The figure shows three views and two pictorial views of one solid part (mm, origin at its lowest corner). Answer the questions. Coordinates: 2 decimals unless noted, no trailing zeros. Order: outer loops, then holes, each group sorted by start corner. A loop starts at its lowest first (then second) coordinate and runs counter-clockwise, first axis right, second up. Notation, with made-up numbers: M -37.75,19.25 L 13.25,19.25 A14 ccw 13.25,33.25 Z; hole C 37,21 d9. An arc over 180 degrees is marked long. Write item = value, one per line. Start each with the question number.
Q1. Find section A-A on z = 3.25. Give the vertices of the cut face in (x, y), and give its area (3 significant figures).
Q2. Straight lines are drawn through the part: line 1 along Y through (x, z) = (36, 11.5); line 2 along X through (y, z) = (64.5, 9.25); line 3 along Y through (x, z) = (5, 7). For each, find the intervals that lie inside material, in ascending order.
Q3. Each of these flat-tipped pins is pushed along its axis until it touches: P1, Ø3, axis at y = 32.5, z = 20.5, coming from the -X side; P2, Ø2, axis at x = 54.5, z = 10.5, coming from the -Y side; P3, Ø4, axis at y = 58.5, z = 8, coming from the -X side. Where does it stop, or does it pass through?
Q4. Determine the mould class of the marked faces 1 and 2 for opening direction X: released by +X, released by -X, zero draft, split by the parting line, or undercut.
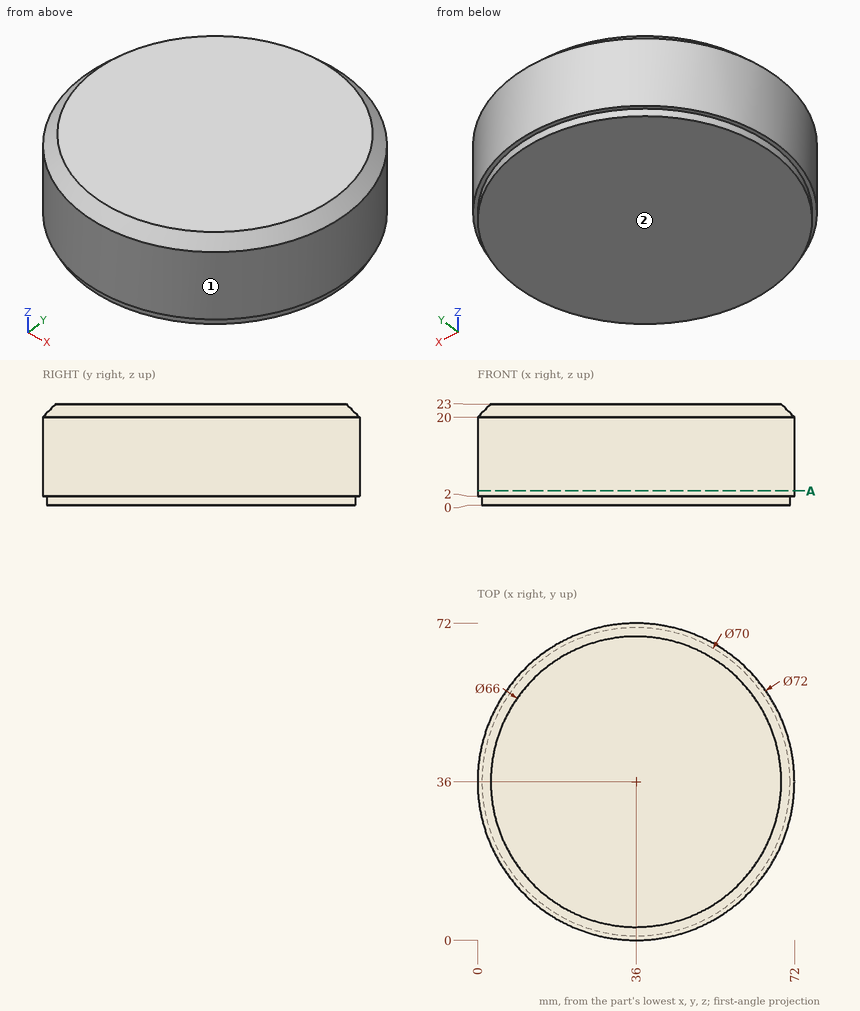
Findings below:
q1.outline = C 36,36 d72
q1.area = 4,070 mm^2
q2.line_1 = 0 to 72
q2.line_2 = 14.01 to 57.99
q2.line_3 = 17.7 to 54.3
q3.P1 = 0.06
q3.P2 = 4.54
q3.P3 = 6.41
q4.face_1 = split by the parting line
q4.face_2 = zero draft
